Build history of the part. All positions in model axes, mm. Round coordinates to 2 decimals unless told otherwise and drop trailing zeros. Loops run counter-clockwise (first coordinate to the right, second up) from the corner with the lowest first, then second, coordinate; pieces in that order, holes last. Notation, with made-up numbers: (72, -1) -> (113, -1) arc R14 cw to (113, 25) -> close; hole circle Ø5 at (45, 14.25). An arc over 180 degrees is marked (long way). Put each result on its own line as item: value. Start each with the question number.
Item 1: Cut at B-B, the plane x = -4.25. List the corners of the cut face in (y, z) (3 decimals), plus the area to 3 significant figures.
Item 2: Cut at C-C, the plane y = 2.75. List the corners of the cut face in (x, z).
Item 3: Drill centre lines: probe 1 along X at (y, z) = (2.5, 1.35); probe 2 along Z at (x, y) = (-2.5, -2.5); probe 3 along Y at (x, z) = (1.25, 2.4). Where is each one in solid material? Low to high. Write a range as [from, to].
Item 4: Cut at A-A, the plane z = 2.25. List the corners of the cut face in (x, y).
```python
from build123d import *

# Parameters (mm, degrees)
SKETCH1_W      = 14.224
SKETCH1_H      = 6.35
EXTRUDE1_DEPTH = 2.54
FILLET1_R      = 0.762
FILLET2_R      = 0.762


with BuildPart() as part:
    # Sketch1 → Extrude1 (new body)
    with BuildSketch(Plane.XY):
        Rectangle(SKETCH1_W, SKETCH1_H)
    extrude(amount=EXTRUDE1_DEPTH)

    # Fillet1
    fillet1_edges = [part.edges().sort_by_distance(p)[0] for p in [
        (7.112, -3.175, 1.27),
        (-7.112, -3.175, 1.27),
        (-7.112, 3.175, 1.27),
        (7.112, 3.175, 1.27),
    ]]
    fillet(fillet1_edges, radius=FILLET1_R)

    # Fillet2
    fillet2_edges = [part.edges().sort_by_distance(p)[0] for p in [
        (0, -3.175, 2.54),
        (-7.112, 0, 2.54),
        (7.112, 0, 2.54),
        (0, 3.175, 2.54),
        (6.888815367, -2.951815367, 2.54),
        (6.888815367, 2.951815367, 2.54),
        (-6.888815367, 2.951815367, 2.54),
        (-6.888815367, -2.951815367, 2.54),
    ]]
    fillet(fillet2_edges, radius=FILLET2_R)


solid = part.part
```
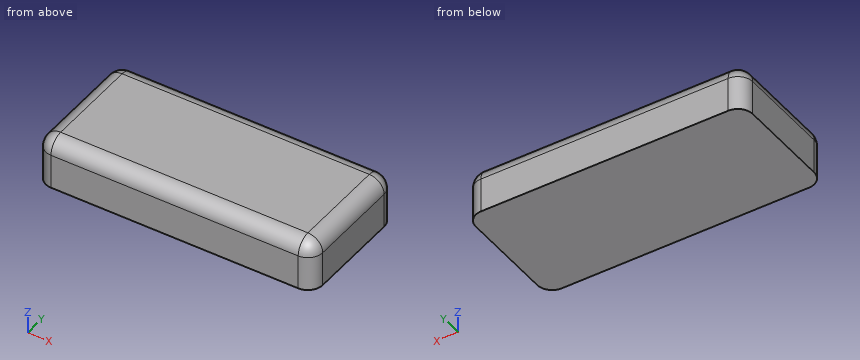
Reply:
1. outline: (-3.175, 0) -> (3.175, 0) -> (3.175, 1.778) arc R0.762 ccw to (2.413, 2.54) -> (-2.413, 2.54) arc R0.762 ccw to (-3.175, 1.778) -> close
1. area: 15.9 mm^2
2. outline: (-7.03, 0) -> (7.03, 0) -> (7.03, 1.78) arc R0.68 ccw to (6.35, 2.46) -> (-6.35, 2.46) arc R0.68 ccw to (-7.03, 1.78) -> close
3. probe 1: x = [-7.11, 7.11]
3. probe 2: z = [0, 2.54]
3. probe 3: y = [-2.85, 2.85]
4. outline: (-6.95, -2.41) arc R0.6 ccw to (-6.35, -3.01) -> (6.35, -3.01) arc R0.6 ccw to (6.95, -2.41) -> (6.95, 2.41) arc R0.6 ccw to (6.35, 3.01) -> (-6.35, 3.01) arc R0.6 ccw to (-6.95, 2.41) -> close
